Autodesk Inventor part; units mm, degrees
ref_plane "YZ Plane" through (0, 0, 0) normal (1, 0, 0) x (0, 1, 0)
ref_plane "XZ Plane" through (0, 0, 0) normal (0, 1, 0) x (-1, 0, 0)
ref_plane "XY Plane" through (0, 0, 0) normal (0, 0, 1) x (1, 0, 0)
sketch "Sketch1" plane through (0, 0, 0) normal (0, 1, 0) x (-1, 0, 0)
  line L0 (0, 0) -> (20, 0)
  line L1 (20, 0) -> (20, -60)
  line L2 (20, -60) -> (0, -60)
  line L3 (0, -60) -> (0, 0)
  dimension "d0" = 60
  dimension "d1" = 20
extrude "Extrusion1" add sketch "Sketch1" along normal blind 16
sketch "Sketch2" plane through (0, 16, 0) normal (0, 1, 0) x (1, 0, 0)
  line L0 (-20, 60) -> (-20, 0)
  line L1 (0, 60) -> (-20, 60)
  point P0 (0, 0)
  point P1 (-10, 30)
  point P2 (-20, 30)
  point P3 (-10, 60)
  dimension "d5" = 10
  dimension "d6" = 30
hole "Hole1" at (-10, 16, -30) direction (0, -1, 0) diameter 6 end through all
fillet "Fillet1" radius 10 4 edges at (-20, 8, 0) (0, 8, 0) (0, 8, -60) (-20, 8, -60)
properties part number "Base_Plate_Spacer_3DPrint"
For this review, take the finished solid that the model builds, in its own axes (mm). Give positions to 0.01 mm unless a question says otherwise; leave off trailing zeros. Write each loop counter-clockwise with the first axis right and the second up, starting at its lowest first coordinate (ties: lowest second). Pieces come first, ordered by that corner, then holes.
Item 1: Take a section at C-C (x = -10.75). Give the boundary of the cut face in (y, z).
Item 2: Insertion check: P1, Ø8, axis at x = -16, y = 3, coming from the +Z side; P2, Ø1, axis at x = -7.5, y = 11, coming from the -Z side; P3, Ø1, axis at x = -13, y = 10, coming from the -Z side. Each pin has a flat end and moves straight along its axis. Give the tip position at first contact, or say it passes through.
Item 3: Wall thickness on probe 1 along X at (y, z) = (10.5, -30); probe 2 along Z at (x, y) = (-10, 7.5); probe 3 along Z at (x, y) = (-8.75, 9.5): over which ranges is each line inside the solid? List them lowest first.
Item 4: Take a section at D-D (x = -3.5). Give the boundary of the cut face in (y, z), and give its area (3 significant figures).
Item 5: Take a section at A-A (z = -30). Give the boundary of the cut face in (x, y).
Item 6: The part is to be moulded in two halves that separate along Z. For faces 1 (the face through (-14, 0, -30)), 2 (the face through (-10, 8, -33)), 3 (the face through (-3.01, 8.11, -2.85)), say which applies: +Z half, -Z half, draft (parallel to the pull), parting line (faces both ways), or undercut.
Established:
1. outline: (0, -59.97) - (16, -59.97) - (16, -32.9) - (0, -32.9) - close; (0, -27.1) - (16, -27.1) - (16, -0.03) - (0, -0.03) - close
2. P1: stops at z = -0.2
2. P2: stops at z = -59.8
2. P3: stops at z = -59.68
3. probe 1: x = -20 to -13, -7 to 0
3. probe 2: z = -60 to -33, -27 to 0
3. probe 3: z = -59.92 to -32.73, -27.27 to -0.08
4. outline: (0, -57.6) - (16, -57.6) - (16, -2.4) - (0, -2.4) - close
4. area: 883 mm2
5. outline: (-20, 0) - (-13, 0) - (-13, 16) - (-20, 16) - close; (-7, 0) - (0, 0) - (0, 16) - (-7, 16) - close
6. face 1: draft
6. face 2: undercut
6. face 3: +Z half
